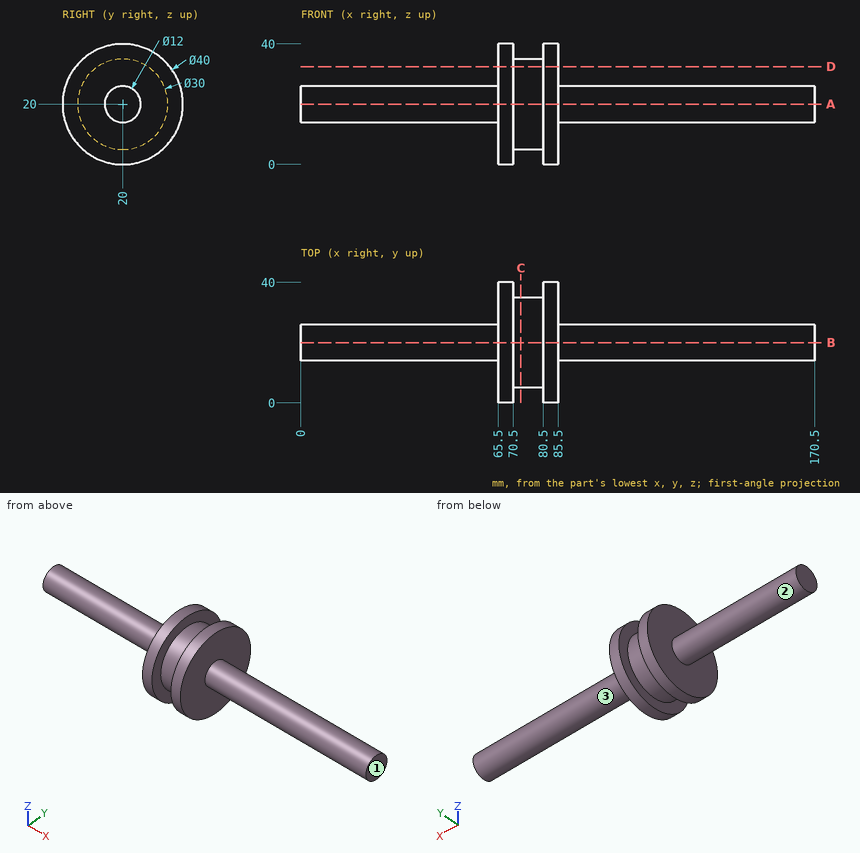
Answer from the drawing. Dimensions are ordinates in mm from the lowest x, y and z of the part. A direction names the side the tool comes from. Coordinates: 2 decimals unless noted, no trailing zeros. Loops run counter-clockwise (first coordinate to the right, second up) from the corner with the lowest first, then second, coordinate; pieces in that order, holes last.
1) Section A-A (z = 20) is taken. Give the vertices of the cut face in (x, y).
Results:
outline: (0, 14) - (65.5, 14) - (65.5, 0) - (70.5, 0) - (70.5, 5) - (80.5, 5) - (80.5, 0) - (85.5, 0) - (85.5, 14) - (170.5, 14) - (170.5, 26) - (85.5, 26) - (85.5, 40) - (80.5, 40) - (80.5, 35) - (70.5, 35) - (70.5, 40) - (65.5, 40) - (65.5, 26) - (0, 26) - close
2) Section C-C (x = 73) is taken. Give the vertices of the cut face in (y, z).
Results:
outline: circle Ø30 at (20, 20)
3) Section D-D (z = 32.5) is taken. Give the vertices of the cut face in (x, y).
Results:
outline: (65.5, 4.39) - (70.5, 4.39) - (70.5, 11.71) - (80.5, 11.71) - (80.5, 4.39) - (85.5, 4.39) - (85.5, 35.61) - (80.5, 35.61) - (80.5, 28.29) - (70.5, 28.29) - (70.5, 35.61) - (65.5, 35.61) - close
4) Consider probe 1 along X at (y, z) = (5.5, 31); probe 2 along X at (y, z) = (12, 15.5); probe 3 along Y at (x, z) = (73, 10.5). Determine where each line is inside the solid, lowest interval first.
Results:
probe 1: x = 65.5 to 70.5, 80.5 to 85.5
probe 2: x = 65.5 to 85.5
probe 3: y = 8.39 to 31.61
5) Flat-ended cylindrical pins translate along their axes: pin 1 (6 mm diameter, centred on x = 27, z = 20.5, fed in from -Y); pin 2 (10 mm diameter, centred on x = 54.5, z = 23, fed in from +Y); pin 3 (4 mm diameter, centred on y = 29.5, z = 19.5, fed in from +X). Find the tip coordinate at first contact, or state that the pin passes through.
Results:
pin 1: stops at y = 14
pin 2: stops at y = 26
pin 3: stops at x = 85.5
6) For the marked faces 1, 2 and 3, determine the directions among +Z, -Z, +X, -X, +Y, -Y from which every point of the face is accessible in a straight line to the end or side of a thin tool.
Results:
face 1: +Z, -Z, +X, +Y, -Y
face 2: -X
face 3: +X
